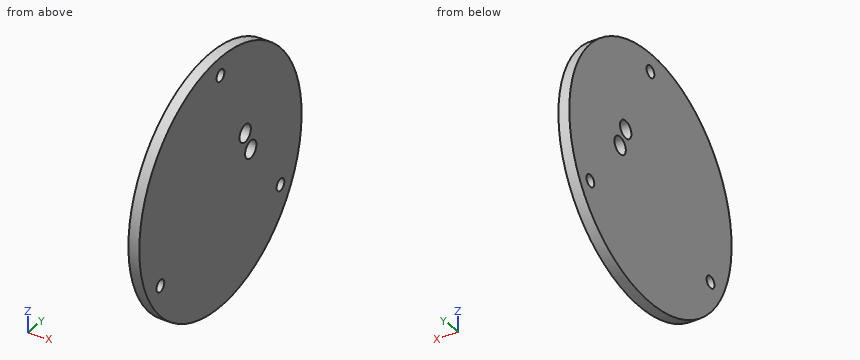
from build123d import *

# Parameters (mm, degrees)
AXIAL_PROFILE_MM_W     = 3
AXIAL_PROFILE_MM_H     = 34.4
AXIAL_HOLES_DEPTH      = 167.945530039
AXIAL_HOLES_DEPTH_BACK = 167.945530039
SKETCH2_R              = 2.4
SKETCH2_R_2            = 1.65


with BuildPart() as part:
    # Axial profile (mm) → Full revolution (revolve)
    with BuildSketch(Plane.XY, mode=Mode.PRIVATE) as full_revolution_sk:
        with Locations((158.2, 17.2)):
            Rectangle(AXIAL_PROFILE_MM_W, AXIAL_PROFILE_MM_H)
    revolve(full_revolution_sk.sketch.rotate(Axis((-110, 0, 0), (1, 0, 0)), 90), axis=Axis((-110, 0, 0), (1, 0, 0)))

    # Sketch2 → Axial holes (cut, two sides: drawn at the far end of the back side and taken through both)
    with BuildSketch(Plane(origin=(0, 0, 0), x_dir=(0, 0, -1), z_dir=(1, 0, 0)).offset(-AXIAL_HOLES_DEPTH_BACK)):
        with Locations((-1.977382665, 12.848733704)):
            Circle(SKETCH2_R)
        with Locations((-7.687206041, 10.483647423)):
            Circle(SKETCH2_R)
        with Locations((-29.4, 0)):
            Circle(SKETCH2_R_2)
        with Locations((14.7, -25.461146871)):
            Circle(SKETCH2_R_2)
        with Locations((14.7, 25.461146871)):
            Circle(SKETCH2_R_2)
    extrude(amount=AXIAL_HOLES_DEPTH + AXIAL_HOLES_DEPTH_BACK, mode=Mode.SUBTRACT)


solid = part.part
The model under review builds one solid part; all positions refer to its coordinate system, in mm. Coordinates: 2 decimals unless noted, no trailing zeros. Loops run counter-clockwise (first coordinate to the right, second up) from the corner with the lowest first, then second, coordinate; pieces in that order, holes last.
(1) Consider section A-A, the plane z = 29. Give the boundary of the cut face in (x, y).
Determined:
outline: (156.7, -18.5) - (159.7, -18.5) - (159.7, -1.6) - (156.7, -1.6) - close; (156.7, 1.6) - (159.7, 1.6) - (159.7, 18.5) - (156.7, 18.5) - close
(2) Consider section C-C, the plane z = -14.7. Give the boundary of the cut face in (x, y), plus the area to 3 significant figures.
Determined:
outline: (156.7, -31.1) - (159.7, -31.1) - (159.7, -27.11) - (156.7, -27.11) - close; (156.7, -23.81) - (159.7, -23.81) - (159.7, 23.81) - (156.7, 23.81) - close; (156.7, 27.11) - (159.7, 27.11) - (159.7, 31.1) - (156.7, 31.1) - close
area: 167 mm2
(3) Consider section D-D, the plane x = 158.4. Give the boundary of the cut face in (y, z).
Determined:
outline: circle Ø68.8 at (0, 0); hole circle Ø3.3 at (-25.46, -14.7); hole circle Ø3.3 at (0, 29.4); hole circle Ø4.8 at (10.48, 7.69); hole circle Ø4.8 at (12.85, 1.98); hole circle Ø3.3 at (25.46, -14.7)
(4) Consider section B-B, the plane y = 0. Give the boundary of the cut face in (x, z), plus the area to 4 significant figures.
Determined:
outline: (156.7, -34.4) - (159.7, -34.4) - (159.7, 27.75) - (156.7, 27.75) - close; (156.7, 31.05) - (159.7, 31.05) - (159.7, 34.4) - (156.7, 34.4) - close
area: 196.5 mm2
(5) Insertion check: P1, Ø1, axis at x = 158.5, z = -5, coming from the +Y side; P2, Ø1.5, axis at x = 158, z = 21.5, coming from the +Y side; P3, Ø2.5, axis at y = 0, z = 29.4, coming from the -X side; P4, Ø1.5, axis at x = 158.5, z = -2, coming from the +Y side. Each pin has a flat end and moves straight along its axis. Give the tip position at first contact, or say it passes through.
Determined:
P1: stops at y = 34.1
P2: stops at y = 27.44
P3: passes through
P4: stops at y = 34.38
(6) Wall thickness on L1, parallel to Y at x = 157.6, z = 8.5; L2, parallel to Y at x = 157.35, z = -1; L3, parallel to Z at x = 156.9, y = 26: over which ranges is each line inside the solid? List them lowest first.
Determined:
L1: y = -33.33 to 8.23, 12.74 to 33.33
L2: y = -34.39 to 34.39
L3: z = -22.52 to -16.26, -13.14 to 22.52
